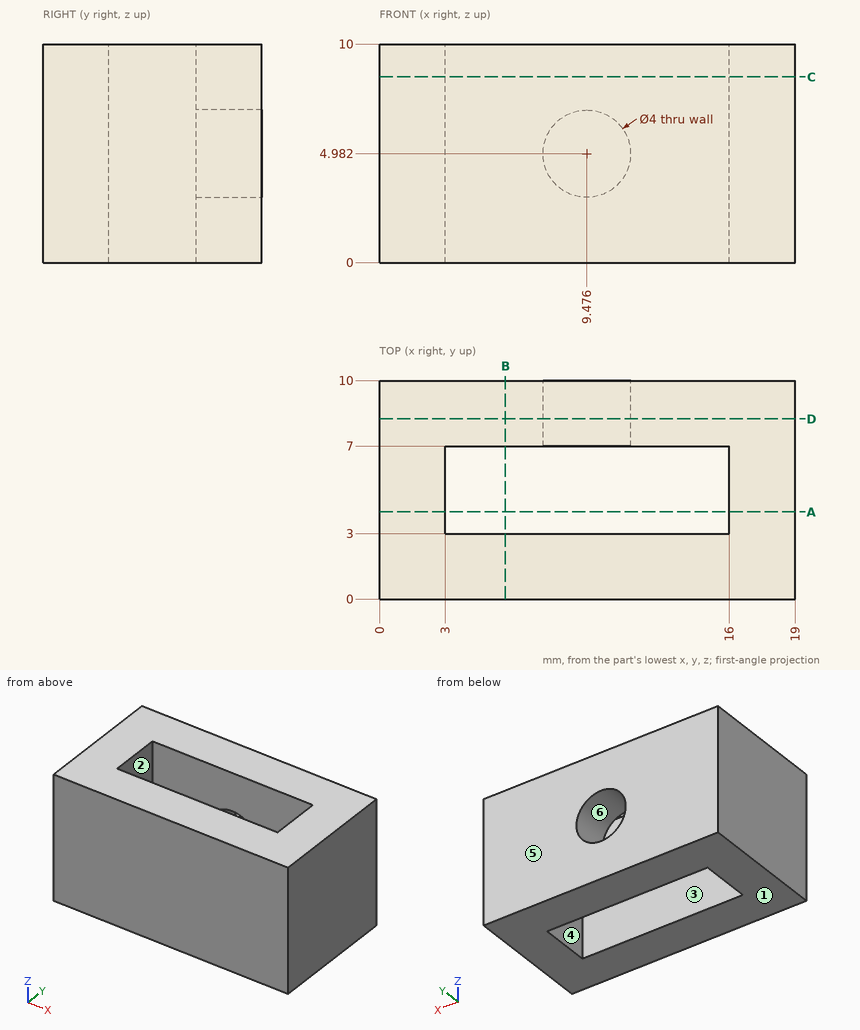
The figure shows three views and two pictorial views of one solid part (mm, origin at its lowest corner). Answer the questions. A direction names the side the tool comes from. Give positions to 0.01 mm unless a question says otherwise; leave off trailing zeros. Write each loop counter-clockwise with the first axis right and the second up, starting at its lowest first coordinate (ties: lowest second). Pieces come first, ordered by that corner, then holes. Notation, with made-up numbers: (4, 84) -> (35, 84) arc R29 ccw to (35, 115) -> close; hole circle Ø3 at (9, -30). An arc over 180 degrees is marked (long way). Answer as a JSON object with one key per item and string values.
1) Section D-D on y = 8.25 is taken. Write down the section's boundary in (x, z).
Findings below:
{"outline": "(0, 0) -> (19, 0) -> (19, 10) -> (0, 10) -> close; hole circle Ø4 at (9.48, 4.98)"}
2) Section C-C on z = 8.5 is taken. Write down the section's boundary in (x, y), then the cut area to 3 significant figures.
Findings below:
{"outline": "(0, 0) -> (19, 0) -> (19, 10) -> (0, 10) -> close; hole (3, 3) -> (16, 3) -> (16, 7) -> (3, 7) -> close", "area": "138 mm^2"}
3) Straight lines are drawn through the part: probe 1 along Y at (x, z) = (15, 5.5); probe 2 along X at (y, z) = (6, 5); probe 3 along Z at (x, y) = (9.75, 8). For each, find the intervals that lie inside material, in ascending order. Write a range as from..to.
Findings below:
{"probe 1": "y = 0..3, 7..10", "probe 2": "x = 0..3, 16..19", "probe 3": "z = 0..3, 6.96..10"}
4) Section A-A on y = 4 is taken. Write down the section's boundary in (x, z).
Findings below:
{"outline": "(0, 0) -> (3, 0) -> (3, 10) -> (0, 10) -> close; (16, 0) -> (19, 0) -> (19, 10) -> (16, 10) -> close"}
5) Section B-B on x = 5.75 is taken. Write down the section's boundary in (y, z), then the cut area to 3 significant figures.
Findings below:
{"outline": "(0, 0) -> (3, 0) -> (3, 10) -> (0, 10) -> close; (7, 0) -> (10, 0) -> (10, 10) -> (7, 10) -> close", "area": "60.0 mm^2"}
6) A tool of negligible diameter and unlimited length cuts with its end or side. For the marked faces 1 and 2, from which of +Z, -Z, +X, -X, +Y, -Y can it reach the whole face along a straight path? Write none if from no direction.
Findings below:
{"face 1": "-Z, +X, -X, +Y, -Y", "face 2": "+Z, -Z"}
7) For a pull along Y with two mould halves and no side action, classify the marked faces 3, 4, 5 and 6 as pulls with the +Y half, pulls with the -Y half, needs draft (parallel to the pull), parting line crosses it, or undercut.
Findings below:
{"face 3": "undercut", "face 4": "undercut", "face 5": "pulls with the +Y half", "face 6": "needs draft"}
8) A flat-ended cylindrical pin translates along its axis: pin 1 Ø6 at (x, y) = (17, 6.5) entering from -Z. Find the tip coordinate at first contact, or state that the pin passes through.
Findings below:
{"pin 1": "stops at z = 0"}
